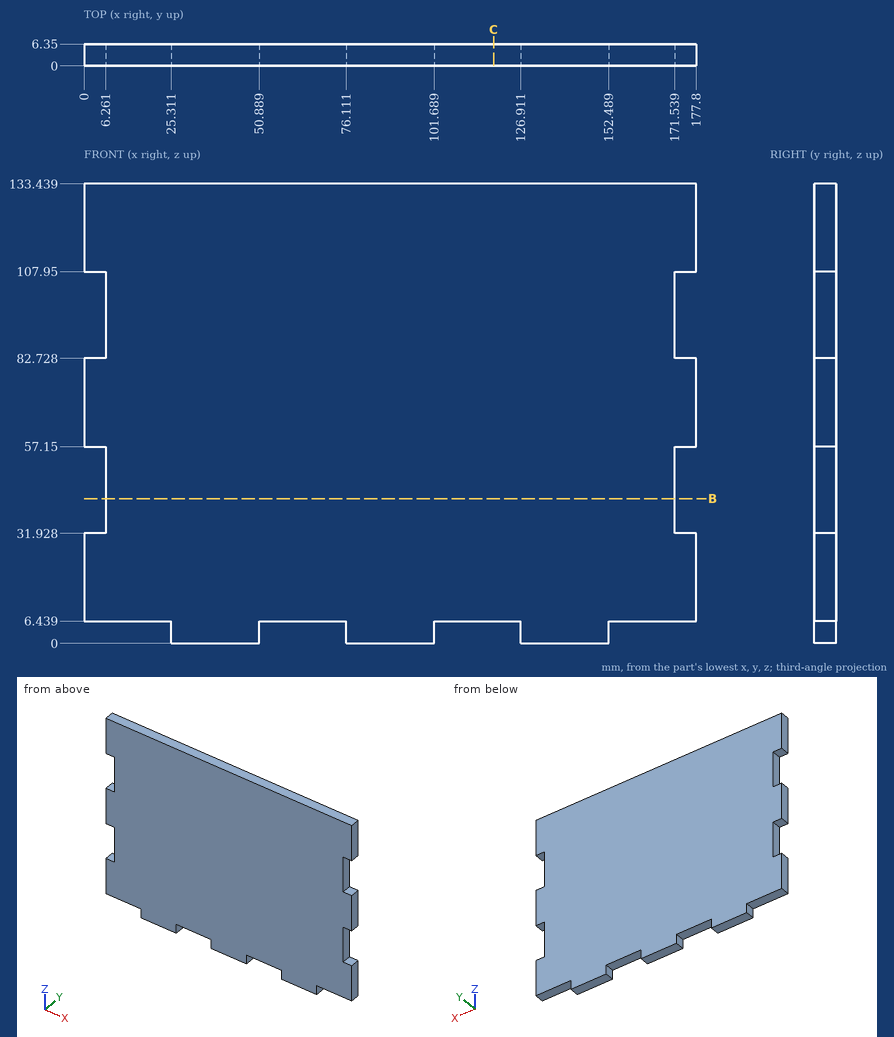
The drawing under review shows one solid part. Ordinate dimensions are in mm from its lowest x, y, z. Round coordinates to 2 decimals unless told otherwise and drop trailing zeros. Loops run counter-clockwise (first coordinate to the right, second up) from the corner with the lowest first, then second, coordinate; pieces in that order, holes last.
Item 1: For line 1 (Z direction, x = 169, y = 1); line 2 (X direction, y = 5.5, z = 86.5), list the stretches that pass through material, from the lowest coordinate up.
Determined:
line 1: z = 6.44 to 133.44
line 2: x = 6.26 to 171.54
Item 2: Clearance check with flat-ended pins moving along their axes: pin 1 Ø3 at (y, z) = (3.5, 4) entering from -X; pin 2 Ø3 at (y, z) = (3.5, 43.5) entering from -X; pin 3 Ø2 at (y, z) = (2, 49.5) entering from +X. State where each tip first meets the part, or that it passes through.
Determined:
pin 1: stops at x = 25.31
pin 2: stops at x = 6.26
pin 3: stops at x = 171.54
Item 3: Take a section at B-B (z = 42). Write out the cut boundary in (x, y).
Determined:
outline: (6.26, 0) - (171.54, 0) - (171.54, 6.35) - (6.26, 6.35) - close
Item 4: Take a section at C-C (x = 119). Write out the cut boundary in (y, z).
Determined:
outline: (0, 6.44) - (6.35, 6.44) - (6.35, 133.44) - (0, 133.44) - close
